Source: CAD feature listing. Evaluate the final solid. Frame: model axes, mm. A direction names the side the tool comes from. Round coordinates to 2 decimals unless told otherwise and drop trailing zeros. Loops run counter-clockwise (first coordinate to the right, second up) from the corner with the lowest first, then second, coordinate; pieces in that order, holes last. Notation, with made-up numbers: (-31, -6.75) - (4, -6.75) arc R17 ccw to (4, 13.25) - close; hole circle Ø8 at (-1, 62). An arc over 180 degrees is marked (long way). One line per question, with ' | ' between items. Start each with the question number.
1. Cut plane C-C (z = -49). Return loops of the section in (x, y).
2. Ray query, line 1 (X direction, y = -8.75, z = 18.5); line 2 (Z direction, x = -9.5, y = -7.75); line 3 (Z direction, x = 23.5, y = -2). Return the intervals inside material, ascending.
3. Cut plane B-B (y = -13.75). Return loops of the section in (x, z).
4. Pin query (flat end, axial travel): pin 1 (10 mm diameter, centred on x = 8.5, z = 30.5, fed in from +Y). Return the tip coordinate at first contact, or that it passes through.
5. Cut plane A-A (x = -22). Return loops of the section in (y, z).
6. Access query for faces 1 (the flat face through (-9, -13, -57.75)), 2 (the flat face through (-1, -12, 55.25)), 3 (the cylindrical face through (29.36, -21.25, -56.48)). Directions: +Z, -Z, +X, -X, +Y, -Y. A direction counts if a zero-diameter tool reaches every point of the face in a straight line with its end or side. Return the directions, or none.
7. Mould query, pull axis X, two halves, no side actions, for faces 4 (the flat face through (38.25, -13, -1)), 5 (the flat face through (-8, -12, -55.25)), 6 (the flat face through (-35.75, -12, -1)), 7 (the flat face through (-37, 0, 5)). Classes: pulls with the +X half, pulls with the -X half, needs draft (parallel to the pull), parting line crosses it, or undercut.
```python
from build123d import *

# Parameters (mm, degrees)
F0_W     = 76.5
F0_H     = 115.5
F1_DEPTH = 26.9
F2_T     = -2.5
F4_DEPTH = 25


with BuildPart() as f1:
    # F0 (on Front) → F1 (new body)
    with BuildSketch(Plane.XZ):
        Rectangle(F0_W, F0_H)
    extrude(amount=F1_DEPTH)

    # F2
    f2_openings = [f1.faces().sort_by_distance(p)[0] for p in [
        (0, 0, 0),
    ]]
    offset(amount=F2_T, openings=f2_openings)

    # F3 (on face) → F4 (cut)
    with BuildSketch(Plane.XY.offset(-55.25)):
        with BuildLine():
            Line((35.75, -15), (35.75, 0))
            Line((35.75, 0), (23.25, 0))
            Line((23.25, 0), (23.25, -15))
            ThreePointArc((23.25, -15), (29.5, -21.25), (35.75, -15))
        make_face()
    extrude(amount=-F4_DEPTH, mode=Mode.SUBTRACT)


solid = f1.part
```
Answers follow:
1) outline: (-38.25, -26.9) - (38.25, -26.9) - (38.25, 0) - (35.75, 0) - (35.75, -24.4) - (-35.75, -24.4) - (-35.75, 0) - (-38.25, 0) - close
2) line 1: x = -38.25 to -35.75, 35.75 to 38.25 | line 2: z = -57.75 to -55.25, 55.25 to 57.75 | line 3: z = 55.25 to 57.75
3) outline: (-38.25, -57.75) - (23.25, -57.75) - (23.25, -55.25) - (-35.75, -55.25) - (-35.75, 55.25) - (35.75, 55.25) - (35.75, -57.75) - (38.25, -57.75) - (38.25, 57.75) - (-38.25, 57.75) - close
4) pin 1: stops at y = -24.4
5) outline: (-26.9, -57.75) - (0, -57.75) - (0, -55.25) - (-24.4, -55.25) - (-24.4, 55.25) - (0, 55.25) - (0, 57.75) - (-26.9, 57.75) - close
6) face 1: -Z, +X, -X, +Y, -Y | face 2: +Y | face 3: -Z, +Y
7) face 4: pulls with the +X half | face 5: undercut | face 6: undercut | face 7: needs draft
